Verification items for the finished model (mm, model axes). Face numbers are marked on the shaded views. A direction names the side the tool comes from. Give positions to 0.01 mm unless a question says otherwise; leave off trailing zeros. Loops run counter-clockwise (first coordinate to the right, second up) from the corner with the lowest first, then second, coordinate; pieces in that order, holes last. Notation, with made-up numbers: (38, -30) -> (67, -30) arc R14 cw to (67, -4) -> close; hole circle Ø5 at (39.25, 54). An arc over 180 degrees is marked (long way). Answer in a Markdown table with one row per item. Add a question column.
Q1. Section check C-C on y = -32. Enter the section's corners in (x, z).
Q2. Gauge pin test, flat ends, axial feed: P1, Ø5, axis at x = -28.5, y = -86.5, coming from the +Z side; P2, Ø6, axis at x = -37.5, z = 32.5, coming from the +Y side; P3, Ø6, axis at x = 8.5, y = -50, coming from the -Z side. Record the tip position at first contact, or that the pin passes through.
Q3. Section check B-B on z = 27. Enter the section's corners in (x, y).
Q4. Section check D-D on x = 34.5. Enter the section's corners in (y, z).
Q5. Set-up check for the marked faces 1 and 2: record each of +Z, -Z, +X, -X, +Y, -Y from which the full face is reachable in a straight line by a thin tool's end or side.
Q6. Material ranges on probe 1 along X at (y, z) = (-20, 23); probe 2 along Z at (x, y) = (-30.5, -30.5); probe 3 along Z at (x, y) = (62.75, -179), recorded low to high.
Q7. Section check A-A on y = -179. Enter the section's corners in (x, z).
```python
from build123d import *

# Parameters (mm, degrees)
F1_DEPTH = 200
F2_SIZE  = 1
F3_R     = 5
F4_DEPTH = 123.2975


with BuildPart() as f1:
    # F0 (on Front) → F1 (new body)
    with BuildSketch(Plane.XZ):
        with BuildLine():
            Line((56.323145, 42.502471), (3.481794, 42.502471))
            Line((3.481794, 42.502471), (-49.359557, 42.502471))
            ThreePointArc((-49.359557, 42.502471), (-55.484592, 40.872204), (-58.166456, 35.129257))
            Line((-58.166456, 35.129257), (-58.166456, 0))
            Line((-58.166456, 0), (-51.817301, 0))
            Line((-51.817301, 0), (-51.817301, 34.510728))
            ThreePointArc((-51.817301, 34.510728), (-50.675188, 36.845939), (-48.130694, 37.378091))
            Line((-48.130694, 37.378091), (3.481794, 37.378091))
            Line((3.481794, 37.378091), (55.094283, 37.378091))
            ThreePointArc((55.094283, 37.378091), (57.638777, 36.845939), (58.78089, 34.510728))
            Line((58.78089, 34.510728), (58.78089, 0))
            Line((58.78089, 0), (65.130044, 0))
            Line((65.130044, 0), (65.130044, 35.129257))
            ThreePointArc((65.130044, 35.129257), (62.448181, 40.872204), (56.323145, 42.502471))
        make_face()
    extrude(amount=F1_DEPTH)

    # F2
    f2_edges = [f1.edges().sort_by_distance(p)[0] for p in [
        (3.481794, -200, 42.502471),
        (3.481794, -200, 37.378091),
        (-55.484592, -200, 40.872204),
        (-50.675188, -200, 36.845939),
        (-51.817301, -200, 17.255364),
        (-58.166456, -200, 17.564629),
        (-54.991878, -200, 0),
        (58.78089, -200, 17.255364),
        (57.638777, -200, 36.845939),
        (62.448181, -200, 40.872204),
        (65.130044, -200, 17.564629),
        (61.955467, -200, 0),
        (58.78089, -100, 0),
        (65.130044, -100, 0),
        (-51.817301, -100, 0),
        (-58.166456, -100, 0),
    ]]
    chamfer(f2_edges, length=F2_SIZE)

    # F3 (on face) → F4 (cut, through all)
    with BuildSketch(Plane(origin=(-58.166456, 0, 0), x_dir=(0, -1, 0), z_dir=(-1, 0, 0))):
        with Locations((179, 19.727895)):
            Circle(F3_R)
    extrude(amount=-F4_DEPTH, mode=Mode.SUBTRACT)


solid = f1.part
```
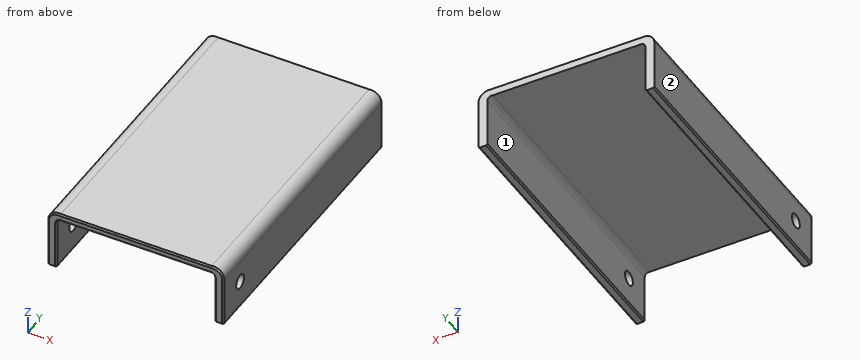
Taken from the geometry:
| question | item | result |
|---|---|---|
| 1 | outline | (-58.17, 1) -> (-57.17, 0) -> (-52.82, 0) -> (-51.82, 1) -> (-51.82, 34.51) arc R2.96 cw to (-48.13, 37.38) -> (55.09, 37.38) arc R2.96 cw to (58.78, 34.51) -> (58.78, 1) -> (59.78, 0) -> (64.13, 0) -> (65.13, 1) -> (65.13, 35.13) arc R7.49 ccw to (56.32, 42.5) -> (-49.36, 42.5) arc R7.49 ccw to (-58.17, 35.13) -> close |
| 2 | P1 | stops at z = 42.5 |
| 2 | P2 | passes through |
| 2 | P3 | stops at z = 37.38 |
| 3 | outline | (-58.17, -199) -> (-57.17, -200) -> (-52.82, -200) -> (-51.82, -199) -> (-51.82, 0) -> (-58.17, 0) -> close; (58.78, -199) -> (59.78, -200) -> (64.13, -200) -> (65.13, -199) -> (65.13, 0) -> (58.78, 0) -> close |
| 4 | outline | (-200, 38.38) -> (-199, 37.38) -> (0, 37.38) -> (0, 42.5) -> (-199, 42.5) -> (-200, 41.5) -> close |
| 5 | face 1 | -Z, +Y, -Y |
| 5 | face 2 | +Z, -Z, -X, +Y, -Y |
| 6 | probe 1 | x = -58.17 to -51.82, 58.78 to 65.13 |
| 6 | probe 2 | z = 37.38 to 42.5 |
| 6 | probe 3 | z = 0 to 14.73, 24.73 to 40.61 |
| 7 | outline | (-58.17, 1) -> (-57.17, 0) -> (-52.82, 0) -> (-51.82, 1) -> (-51.82, 14.73) -> (-58.17, 14.73) -> close; (-58.17, 24.73) -> (-51.82, 24.73) -> (-51.82, 34.51) arc R2.96 cw to (-48.13, 37.38) -> (55.09, 37.38) arc R2.96 cw to (58.78, 34.51) -> (58.78, 24.73) -> (65.13, 24.73) -> (65.13, 35.13) arc R7.49 ccw to (56.32, 42.5) -> (-49.36, 42.5) arc R7.49 ccw to (-58.17, 35.13) -> close; (58.78, 1) -> (59.78, 0) -> (64.13, 0) -> (65.13, 1) -> (65.13, 14.73) -> (58.78, 14.73) -> close |
